Here's how the part is built. I have some questions about the finished solid (model axes, mm). Face numbers are marked on the shaded views. A direction names the side the tool comes from. Coordinates: 2 decimals unless noted, no trailing zeros. Loops run counter-clockwise (first coordinate to the right, second up) from the corner with the lowest first, then second, coordinate; pieces in that order, holes last. Notation, with made-up numbers: M -14,72 L 31,72 A22 ccw 31,105 Z; hole C 88.25,32 d2. An arc over 180 degrees is marked long. Use CSV: the item, a comma, the result in double quotes. Start each with the question number.
Q1. If we section it at D-D (y = 0): Please give me the cut outline in (x, z).
Q2. If we section it at A-A (z = -4): State how many separate pieces and enclosed holes the cut face has, and give its area (3 significant figures).
Q3. If we mould it in two halves opening along Y, with no side actions, what happens to the marked faces 6, 7 and 8? For each: +Y half, -Y half, draft (parallel to the pull), parting line (faces both ways), or undercut.
Q4. Which directions (+Z, -Z, +X, -X, +Y, -Y) give clear straight access to the entire face, cutting with the end or side of a thin tool? Please do the marked faces 1, 2, 3, 4 and 5.
Q5. For pin 1 Ø1 at (y, z) = (8.5, -3.5) entering from +X; pin 2 Ø4.5 at (x, y) = (0, 0) entering from -Z; pin 3 Ø0.6 at (x, y) = (9.5, -5) entering from -Z, each with a flat end and sliding along its axis, tell me the tip position at first contact or that it passes through.
Q6. If we section it at C-C (x = -13): Please give me the cut outline in (y, z) (3 decimals).
Q7. Please list where these lines run through material, in increasing order: probe 1 along Y at (x, z) = (-13, -4.4) (3 decimals); probe 2 along Y at (x, z) = (9.5, 2); probe 3 along X at (y, z) = (4.55, 1.25). Write a range as [from, to].
Q8. If we section it at B-B (z = 4.25): Please give me the cut outline in (x, y), and give its area (3 significant figures).
from build123d import *

# Parameters (mm, degrees)
BOSS_EXTRUDE1_DEPTH     = 1
SKETCH2_R               = 1.51
BOSS_EXTRUDE2_DEPTH     = 5.5
SKETCH3_R               = 3.5
BOSS_EXTRUDE3_DEPTH     = 1
SKETCH4_W               = 2
SKETCH4_H               = 17
BOSS_EXTRUDE4_DEPTH     = 6
SKETCH5_W               = 18
SKETCH5_H               = 2
BOSS_EXTRUDE5_DEPTH     = 6
SKETCH6_W               = 7
SKETCH6_H               = 2
BOSS_EXTRUDE6_DEPTH     = 5
BOSS_EXTRUDE7_DEPTH     = 6
CUT_EXTRUDE1_DEPTH      = 21.639767441
SKETCH9_W               = 2.937742252
SKETCH9_H               = 8
CUT_EXTRUDE2_DEPTH      = 6
CUT_EXTRUDE11_START     = -6
SKETCH21_R              = 9.25
SKETCH21_R_2            = 3.5
CUT_EXTRUDE11_DEPTH     = 6
SKETCH10_W              = 32
SKETCH10_H              = 2
BOSS_EXTRUDE8_DEPTH     = 7
FILLET1_R               = 0.5
SKETCH11_R              = 0.625
BOSS_EXTRUDE9_DEPTH     = 2
SKETCH14_W              = 3.5
SKETCH14_H              = 2
CUT_EXTRUDE5_DEPTH      = 24.937418532
SKETCH12_R              = 0.675
CUT_EXTRUDE3_DEPTH      = 2.5
CUT_EXTRUDE6_DEPTH      = 2
FILLET2_R               = 0.5
FILLET3_R               = 0.5
FILLET4_R               = 2
CUT_EXTRUDE7_DEPTH      = 25.677925456
CUT_EXTRUDE7_DEPTH_BACK = 1
SKETCH19_R              = 0.25
CUT_EXTRUDE9_DEPTH      = 2
SKETCH20_W              = 2
SKETCH20_H              = 3
CUT_EXTRUDE10_DEPTH     = 24.937418532


with BuildPart() as part:
    # Sketch1 → Boss-Extrude1 (new body)
    with BuildSketch(Plane.XY):
        Polygon((-11, 6), (-11, 11), (11, 11), (11, 6), (11, -6), (-11, -6), align=None)
    extrude(amount=BOSS_EXTRUDE1_DEPTH)

    # Sketch2 → Boss-Extrude2 (add)
    with BuildSketch(Plane(origin=(0, 0, 0), x_dir=(-1, 0, 0), z_dir=(0, 0, -1))):
        with Locations(Location((0, 0, 0), (0, 0, 180))):
            Circle(SKETCH2_R)
    extrude(amount=BOSS_EXTRUDE2_DEPTH)

    # Sketch3 → Boss-Extrude3 (add)
    with BuildSketch(Plane(origin=(0, 0, 0), x_dir=(-1, 0, 0), z_dir=(0, 0, -1))):
        with Locations(Location((0, 0, 0), (0, 0, 180))):
            Circle(SKETCH3_R)
    extrude(amount=BOSS_EXTRUDE3_DEPTH)

    # Sketch4 → Boss-Extrude4 (add)
    with BuildSketch(Plane(origin=(0, 0, 0), x_dir=(-1, 0, 0), z_dir=(0, 0, -1))):
        with Locations((10, 2.5)):
            Rectangle(SKETCH4_W, SKETCH4_H)
        with Locations((-10, 2.5)):
            Rectangle(SKETCH4_W, SKETCH4_H)
    extrude(amount=BOSS_EXTRUDE4_DEPTH)

    # Sketch5 → Boss-Extrude5 (add)
    with BuildSketch(Plane(origin=(0, 0, 0), x_dir=(-1, 0, 0), z_dir=(0, 0, -1))):
        with Locations((0, 10)):
            Rectangle(SKETCH5_W, SKETCH5_H)
    extrude(amount=BOSS_EXTRUDE5_DEPTH)

    # Sketch6 → Boss-Extrude6 (add)
    with BuildSketch(Plane(origin=(11, 0, 0), x_dir=(0, 0, -1), z_dir=(1, 0, 0))):
        with Locations((2.5, -5)):
            Rectangle(SKETCH6_W, SKETCH6_H)
        with Locations((2.5, 5)):
            Rectangle(SKETCH6_W, SKETCH6_H)
    boss_extrude6 = extrude(amount=BOSS_EXTRUDE6_DEPTH)

    # Mirror1: Boss-Extrude6 across plane
    add(boss_extrude6.mirror(Plane(origin=(0, 0, 0), x_dir=(0, 0, 1), z_dir=(1, 0, 0))))

    # Sketch7 → Boss-Extrude7 (add)
    with BuildSketch(Plane(origin=(0, 0, -6), x_dir=(-1, 0, 0), z_dir=(0, 0, -1))):
        with BuildLine():
            ThreePointArc((-6.708203932, -6), (-8.407551231, -3.211398808), (-9, 0))
            Line((-9, 0), (-9, -6))
            Line((-9, -6), (-6.708203932, -6))
        make_face()
        with BuildLine():
            Line((-9, 9), (-9, 0))
            ThreePointArc((-9, 0), (-6.363961031, 6.363961031), (0, 9))
            Line((0, 9), (-9, 9))
        make_face()
    boss_extrude7 = extrude(amount=-BOSS_EXTRUDE7_DEPTH)

    # Sketch8 → Cut-Extrude1 (cut, through all)
    with BuildSketch(Plane(origin=(0, 0, -6), x_dir=(-1, 0, 0), z_dir=(0, 0, -1))):
        with BuildLine():
            Line((-11, 4), (-8.61684397, 4))
            ThreePointArc((-8.61684397, 4), (-9.5, 0), (-8.61684397, -4))
            Line((-8.61684397, -4), (-11, -4))
            Line((-11, -4), (-11, 4))
        make_face()
    cut_extrude1 = extrude(amount=-CUT_EXTRUDE1_DEPTH, mode=Mode.SUBTRACT)

    # Sketch9 → Cut-Extrude2 (cut)
    with BuildSketch(Plane(origin=(0, 0, -6), x_dir=(-1, 0, 0), z_dir=(0, 0, -1))):
        with Locations((-9.531128874, 0)):
            Rectangle(SKETCH9_W, SKETCH9_H)
    cut_extrude2 = extrude(amount=-CUT_EXTRUDE2_DEPTH, mode=Mode.SUBTRACT)

    # Mirror2: Boss-Extrude7, Cut-Extrude1, Cut-Extrude2 across plane
    add(boss_extrude7.mirror(Plane(origin=(0, 0, 0), x_dir=(0, 0, 1), z_dir=(1, 0, 0))))
    add(cut_extrude1.mirror(Plane(origin=(0, 0, 0), x_dir=(0, 0, 1), z_dir=(1, 0, 0))), mode=Mode.SUBTRACT)
    add(cut_extrude2.mirror(Plane(origin=(0, 0, 0), x_dir=(0, 0, 1), z_dir=(1, 0, 0))), mode=Mode.SUBTRACT)

    # Sketch21 → Cut-Extrude11 (cut)
    with BuildSketch(Plane(origin=(0, 0, -6), x_dir=(-1, 0, 0), z_dir=(0, 0, -1)).offset(CUT_EXTRUDE11_START)):
        Circle(SKETCH21_R)
        with Locations(Location((0, 0, 0), (0, 0, 180))):
            Circle(SKETCH21_R_2, mode=Mode.SUBTRACT)
    extrude(amount=CUT_EXTRUDE11_DEPTH, mode=Mode.SUBTRACT)

    # Sketch10 → Boss-Extrude8 (add)
    with BuildSketch(Plane.XY.offset(1)):
        with Locations((0, -5)):
            Rectangle(SKETCH10_W, SKETCH10_H)
        with Locations((0, 5)):
            Rectangle(SKETCH10_W, SKETCH10_H)
    extrude(amount=BOSS_EXTRUDE8_DEPTH)

    # Fillet1
    fillet1_edges = [part.edges().sort_by_distance(p)[0] for p in [
        (9.5, 0, 1),
        (-9.5, 0, 1),
    ]]
    fillet(fillet1_edges, radius=FILLET1_R)

    # Sketch11 → Boss-Extrude9 (add)
    with BuildSketch(Plane(origin=(0, 0, -6), x_dir=(-1, 0, 0), z_dir=(0, 0, -1))):
        with Locations(Location((-13, -5, 0), (0, 0, 180))):
            Circle(SKETCH11_R)
    boss_extrude9 = extrude(amount=BOSS_EXTRUDE9_DEPTH)

    # Sketch14 → Cut-Extrude5 (cut, through all)
    with BuildSketch(Plane(origin=(0, 0, -6), x_dir=(-1, 0, 0), z_dir=(0, 0, -1))):
        with Locations((9.25, 7)):
            Rectangle(SKETCH14_W, SKETCH14_H)
        with Locations((-9.25, 7)):
            Rectangle(SKETCH14_W, SKETCH14_H)
    extrude(amount=-CUT_EXTRUDE5_DEPTH, mode=Mode.SUBTRACT)

    # Sketch12 → Cut-Extrude3 (cut)
    with BuildSketch(Plane(origin=(0, 0, -6), x_dir=(-1, 0, 0), z_dir=(0, 0, -1))):
        with Locations((13, -5)):
            Circle(SKETCH12_R)
    cut_extrude3 = extrude(amount=-CUT_EXTRUDE3_DEPTH, mode=Mode.SUBTRACT)

    # Sketch16 → Cut-Extrude6 (cut)
    with BuildSketch(Plane(origin=(0, 6, 0), x_dir=(1, 0, 0), z_dir=(0, 1, 0))):
        with BuildLine():
            Line((-7.5, 0), (-7.5, -1))
            ThreePointArc((-7.5, -1), (-7.25, -0.5), (-7.5, 0))
        make_face()
    cut_extrude6 = extrude(amount=CUT_EXTRUDE6_DEPTH, mode=Mode.SUBTRACT)

    # Mirror3: Boss-Extrude9, Cut-Extrude3 across plane
    add(boss_extrude9.mirror(Plane.ZX))
    add(cut_extrude3.mirror(Plane.ZX), mode=Mode.SUBTRACT)

    # Mirror4: Cut-Extrude6 across plane
    add(cut_extrude6.mirror(Plane(origin=(0, 0, 0), x_dir=(0, 0, 1), z_dir=(1, 0, 0))), mode=Mode.SUBTRACT)

    # Fillet2
    fillet2_edges = [part.edges().sort_by_distance(p)[0] for p in [
        (12.375, -5, -6),
        (12.375, 5, -6),
    ]]
    fillet(fillet2_edges, radius=FILLET2_R)

    # Fillet3
    # the kernel refuses this fillet: 0.5 mm, written as the material it takes off along each edge
    with BuildSketch(Plane(origin=(-13, -5, -6), x_dir=(-1, 0, 0), z_dir=(0, -1, 0))) as fillet3_piece_1:
        with BuildLine():
            CenterArc((0.675 + FILLET3_R, -FILLET3_R), FILLET3_R, 90, 90)
            Line((0.675, -FILLET3_R), (0.675, 0))
            Line((0.675, 0), (0.675 + FILLET3_R, 0))
        make_face()
    revolve(axis=Axis((-13, -5, -6), (0, 0, -1)), mode=Mode.SUBTRACT)
    with BuildSketch(Plane(origin=(-13, 5, -6), x_dir=(-1, 0, 0), z_dir=(0, 1, 0))) as fillet3_piece_2:
        with BuildLine():
            CenterArc((0.675 + FILLET3_R, FILLET3_R), FILLET3_R, 180, 90)
            Line((0.675, FILLET3_R), (0.675, 0))
            Line((0.675, 0), (0.675 + FILLET3_R, 0))
        make_face()
    revolve(axis=Axis((-13, 5, -6), (0, 0, 1)), mode=Mode.SUBTRACT)

    # Fillet4
    fillet4_edges = [part.edges().sort_by_distance(p)[0] for p in [
        (16, -5, 8),
        (-16, -5, 8),
        (-16, 5, 8),
        (16, 5, 8),
    ]]
    fillet(fillet4_edges, radius=FILLET4_R)

    # Sketch17 → Cut-Extrude7 (cut, two sides: drawn at the far end of the back side and taken through both)
    with BuildSketch(Plane.XZ.offset(6).offset(-CUT_EXTRUDE7_DEPTH_BACK)):
        with BuildLine():
            Line((-16, 6), (-16, -6))
            Line((-16, -6), (-14.5, -6))
            Line((-14.5, -6), (-14.5, 6))
            ThreePointArc((-14.5, 6), (-14.353553391, 6.353553391), (-14, 6.5))
            Line((-14, 6.5), (14, 6.5))
            ThreePointArc((14, 6.5), (14.353553391, 6.353553391), (14.5, 6))
            Line((14.5, 6), (14.5, -6))
            Line((14.5, -6), (16, -6))
            Line((16, -6), (16, 6))
            ThreePointArc((16, 6), (15.414213562, 7.414213562), (14, 8))
            Line((14, 8), (-14, 8))
            ThreePointArc((-14, 8), (-15.414213562, 7.414213562), (-16, 6))
        make_face()
    extrude(amount=CUT_EXTRUDE7_DEPTH + CUT_EXTRUDE7_DEPTH_BACK, mode=Mode.SUBTRACT)

    # Sketch19 → Cut-Extrude9 (cut)
    with BuildSketch(Plane(origin=(0, 6, 0), x_dir=(1, 0, 0), z_dir=(0, 1, 0))):
        with Locations(Location((0, -1.25, 0), (0, 0, 90))):
            Circle(SKETCH19_R)
        with Locations(Location((0, -7.25, 0), (0, 0, 270))):
            Circle(SKETCH19_R)
    extrude(amount=-CUT_EXTRUDE9_DEPTH, mode=Mode.SUBTRACT)

    # Sketch20 → Cut-Extrude10 (cut, through all)
    with BuildSketch(Plane(origin=(0, 0, -6), x_dir=(-1, 0, 0), z_dir=(0, 0, -1))):
        with Locations((-10, 9.5)):
            Rectangle(SKETCH20_W, SKETCH20_H)
        with Locations((10, 9.5)):
            Rectangle(SKETCH20_W, SKETCH20_H)
    extrude(amount=-CUT_EXTRUDE10_DEPTH, mode=Mode.SUBTRACT)


solid = part.part
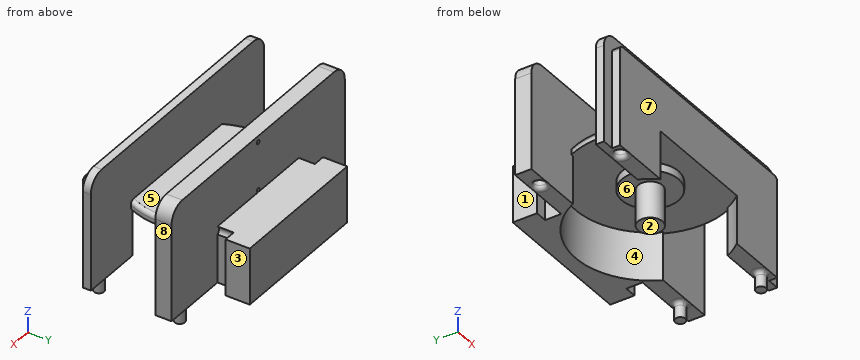
Results below:
1,outline,"M -9.5,0 L -3.5,0 L -3.5,-1 L -1.51,-1 L -1.51,-5.5 L 1.51,-5.5 L 1.51,-1 L 3.5,-1 L 3.5,0 L 9.5,0 L 9.5,0.5 A0.5 ccw 9,1 L -9,1 A0.5 ccw -9.5,0.5 Z"
2,separate pieces,"4"
2,enclosed holes,"2"
2,area,"120 mm^2"
3,face 6,"undercut"
3,face 7,"-Y half"
3,face 8,"draft"
4,face 1,"+Z, -Z, -X, +Y"
4,face 2,"-Z, +X, -X, -Y"
4,face 3,"+Z, -Z, +X, +Y"
4,face 4,"-Z"
4,face 5,"+Z, +X, -X"
5,pin 1,"x = 9"
5,pin 2,"z = -5.5"
5,pin 3,"z = -6"
6,outline,"M -6,-5.968 A0.5 ccw -5.675,-5.5 L -5.675,-3.5 L -4.325,-3.5 L -4.325,-5.5 A0.5 ccw -4,-5.968 L -4,8 L -5,8 L -5,6.5 L -6,6.5 Z; M 4,-5.968 A0.5 ccw 4.325,-5.5 L 4.325,-3.5 L 5.675,-3.5 L 5.675,-5.5 A0.5 ccw 6,-5.968 L 6,8 L 4,8 Z"
7,probe 1,"[-6, -5.675], [-4.325, -4], [4, 4.325], [5.675, 6]"
7,probe 2,"[-6, -4], [4, 6]"
7,probe 3,"[-16, -0.25], [0.25, 16]"
8,outline,"M -16,-5 L -14.5,-5 L -14.5,-6 L 14.5,-6 L 14.5,-5 L 16,-5 L 16,-4 L -16,-4 Z; M -16,4 L 16,4 L 16,6 L -16,6 Z"
8,area,"125 mm^2"
